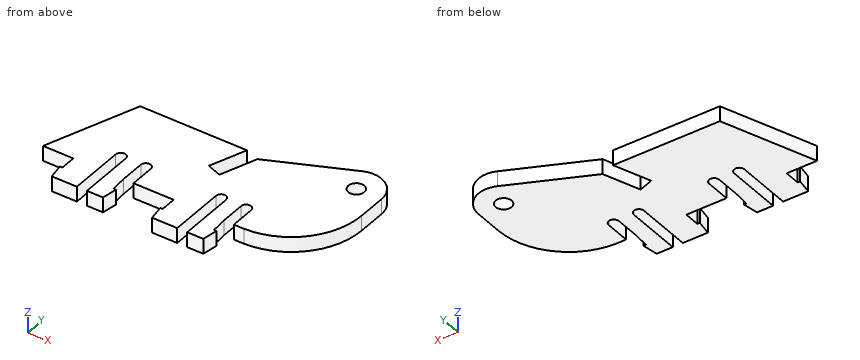
from build123d import *

# Parameters (mm, degrees)
SKETCH1_R           = 1.5875
BOSS_EXTRUDE1_DEPTH = 3
TABS_DEPTH          = 3
TAB_RELIEF_REACH    = 195.217


with BuildPart() as part:
    # Sketch1 → Boss-Extrude1 (new body)
    with BuildSketch(Plane.XY):
        with BuildLine():
            Line((-44.534658728, 169.908603759), (-60.444091073, 162.821196289))
            Line((-60.444091073, 162.821196289), (-63.031525128, 155.712279649))
            Line((-63.031525128, 155.712279649), (-65.85060299, 156.738340079))
            Line((-65.85060299, 156.738340079), (-63.263168935, 163.847256719))
            Line((-63.263168935, 163.847256719), (-84.546724385, 163.847256719))
            Line((-84.546724385, 163.847256719), (-91.147316237, 145.712279649))
            Line((-91.147316237, 145.712279649), (-51.5, 145.712279649))
            ThreePointArc((-51.5, 145.712279649), (-41.600505063, 149.812784712), (-37.5, 159.712279649))
            Line((-37.5, 159.712279649), (-37.5, 165.341310922))
            ThreePointArc((-37.5, 165.341310922), (-39.777252641, 169.534954543), (-44.534658728, 169.908603759))
        make_face()
        with Locations((-42.5, 165.341310922)):
            Circle(SKETCH1_R, mode=Mode.SUBTRACT)
    extrude(amount=BOSS_EXTRUDE1_DEPTH)

    # Sketch3 → tabs (add)
    with BuildSketch(Plane(origin=(0, 0, 0), x_dir=(-1, 0, 0), z_dir=(0, 0, -1))):
        with BuildLine():
            Line((54.9, 142.612279649), (55.1, 145.712279649))
            Line((55.1, 145.712279649), (55.1, 150.612279649))
            ThreePointArc((55.1, 150.612279649), (54.1, 151.612279649), (53.1, 150.612279649))
            Line((53.1, 150.612279649), (53.1, 145.712279649))
            Line((53.1, 145.712279649), (51.1, 145.712279649))
            Line((51.1, 145.712279649), (51.1, 152.712279649))
            Line((51.1, 152.712279649), (67.1, 152.712279649))
            Line((67.1, 152.712279649), (67.1, 145.712279649))
            Line((67.1, 145.712279649), (65.1, 145.712279649))
            Line((65.1, 145.712279649), (65.1, 142.612279649))
            Line((65.1, 142.612279649), (65.6, 142.612279649))
            Line((65.6, 142.612279649), (65.1, 139.612279649))
            Line((65.1, 139.612279649), (60.1, 139.612279649))
            Line((60.1, 139.612279649), (60.1, 150.612279649))
            ThreePointArc((60.1, 150.612279649), (59.1, 151.612279649), (58.1, 150.612279649))
            Line((58.1, 150.612279649), (58.1, 139.612279649))
            Line((58.1, 139.612279649), (54.9, 139.612279649))
            Line((54.9, 139.612279649), (54.4, 142.612279649))
            Line((54.4, 142.612279649), (54.9, 142.612279649))
        make_face()
        with BuildLine():
            Line((74.9, 142.612279649), (75.1, 145.712279649))
            Line((75.1, 145.712279649), (75.1, 150.612279649))
            ThreePointArc((75.1, 150.612279649), (74.1, 151.612279649), (73.1, 150.612279649))
            Line((73.1, 150.612279649), (73.1, 145.712279649))
            Line((73.1, 145.712279649), (71.1, 145.712279649))
            Line((71.1, 145.712279649), (71.1, 152.712279649))
            Line((71.1, 152.712279649), (87.1, 152.712279649))
            Line((87.1, 152.712279649), (87.1, 145.712279649))
            Line((87.1, 145.712279649), (85.1, 145.712279649))
            Line((85.1, 145.712279649), (85.1, 142.612279649))
            Line((85.1, 142.612279649), (85.6, 142.612279649))
            Line((85.6, 142.612279649), (85.1, 139.612279649))
            Line((85.1, 139.612279649), (80.1, 139.612279649))
            Line((80.1, 139.612279649), (80.1, 150.612279649))
            ThreePointArc((80.1, 150.612279649), (79.1, 151.612279649), (78.1, 150.612279649))
            Line((78.1, 150.612279649), (78.1, 139.612279649))
            Line((78.1, 139.612279649), (74.9, 139.612279649))
            Line((74.9, 139.612279649), (74.4, 142.612279649))
            Line((74.4, 142.612279649), (74.9, 142.612279649))
        make_face()
    extrude(amount=-TABS_DEPTH)

    # Sketch4 → tab relief (cut, up to next)
    with BuildSketch(Plane(origin=(0, 0, 0), x_dir=(-1, 0, 0), z_dir=(0, 0, -1)), mode=Mode.PRIVATE) as tab_relief_sk1:
        with BuildLine():
            Line((55.1, 145.712279649), (55.1, 150.612279649))
            ThreePointArc((55.1, 150.612279649), (54.1, 151.612279649), (53.1, 150.612279649))
            Line((53.1, 150.612279649), (53.1, 145.712279649))
            Line((53.1, 145.712279649), (55.1, 145.712279649))
        make_face()
    tab_relief_tool1 = extrude(tab_relief_sk1.sketch, amount=-TAB_RELIEF_REACH, mode=Mode.PRIVATE) & part.part
    # Sketch4 → tab relief (cut, up to next)
    with BuildSketch(Plane(origin=(0, 0, 0), x_dir=(-1, 0, 0), z_dir=(0, 0, -1)), mode=Mode.PRIVATE) as tab_relief_sk2:
        with BuildLine():
            Line((75.1, 145.712279649), (75.1, 150.612279649))
            ThreePointArc((75.1, 150.612279649), (74.1, 151.612279649), (73.1, 150.612279649))
            Line((73.1, 150.612279649), (73.1, 145.712279649))
            Line((73.1, 145.712279649), (75.1, 145.712279649))
        make_face()
    tab_relief_tool2 = extrude(tab_relief_sk2.sketch, amount=-TAB_RELIEF_REACH, mode=Mode.PRIVATE) & part.part
    # Sketch4 → tab relief (cut, up to next)
    with BuildSketch(Plane(origin=(0, 0, 0), x_dir=(-1, 0, 0), z_dir=(0, 0, -1)), mode=Mode.PRIVATE) as tab_relief_sk3:
        with BuildLine():
            Line((58.1, 150.612279649), (58.1, 145.712279649))
            Line((58.1, 145.712279649), (60.1, 145.712279649))
            Line((60.1, 145.712279649), (60.1, 150.612279649))
            ThreePointArc((60.1, 150.612279649), (59.1, 151.612279649), (58.1, 150.612279649))
        make_face()
    tab_relief_tool3 = extrude(tab_relief_sk3.sketch, amount=-TAB_RELIEF_REACH, mode=Mode.PRIVATE) & part.part
    # Sketch4 → tab relief (cut, up to next)
    with BuildSketch(Plane(origin=(0, 0, 0), x_dir=(-1, 0, 0), z_dir=(0, 0, -1)), mode=Mode.PRIVATE) as tab_relief_sk4:
        with BuildLine():
            Line((78.1, 150.612279649), (78.1, 145.712279649))
            Line((78.1, 145.712279649), (80.1, 145.712279649))
            Line((80.1, 145.712279649), (80.1, 150.612279649))
            ThreePointArc((80.1, 150.612279649), (79.1, 151.612279649), (78.1, 150.612279649))
        make_face()
    tab_relief_tool4 = extrude(tab_relief_sk4.sketch, amount=-TAB_RELIEF_REACH, mode=Mode.PRIVATE) & part.part
    add(tab_relief_tool1.solids().sort_by_distance((-54.1, 148.55936, 0))[0], mode=Mode.SUBTRACT)
    add(tab_relief_tool2.solids().sort_by_distance((-74.1, 148.55936, 0))[0], mode=Mode.SUBTRACT)
    add(tab_relief_tool3.solids().sort_by_distance((-59.1, 148.55936, 0))[0], mode=Mode.SUBTRACT)
    add(tab_relief_tool4.solids().sort_by_distance((-79.1, 148.55936, 0))[0], mode=Mode.SUBTRACT)


solid = part.part
Can you work these out from the model? Positions are in its coordinate system, mm. Coordinates: 2 decimals unless noted, no trailing zeros. Loops run counter-clockwise (first coordinate to the right, second up) from the corner with the lowest first, then second, coordinate; pieces in that order, holes last. Notation, with made-up numbers: (15.5, 17.5) - (57.5, 17.5) arc R10 ccw to (57.5, 26.5) - close; hole circle Ø9 at (65, 34). An arc over 180 degrees is marked (long way). Answer as a JSON object with one key per item and string values. Group by question number.
Item 1: If we section it at C-C (x = -67.5): List the corners of the cut face in (y, z) for me, plus the area to 3 significant figures.
Item 2: For pin 1 (1.5 mm diameter, centred on y = 146.5, z = 1, fed in from +X); pin 2 (1.5 mm diameter, centred on y = 143.5, z = 1.5, fed in from -X); pin 3 (1 mm diameter, centred on x = -52, z = 1, fed in from -Y), each with a flat end and sliding along its axis, tell me the tip position at first contact or that it passes through.
Item 3: If we section it at A-A (x = -42.5): List the corners of the cut face in (y, z) for me, plus the area to 3 significant figures.
Item 4: If we section it at B-B (y = 147): List the corners of the cut face in (x, z) for me.
Item 5: If we section it at D-D (y = 154): List the corners of the cut face in (x, z) for me.
Item 6: If I drill on L1, parallel to X at y = 145.5, z = 2.5; L2, parallel to X at y = 151.5, z = 2.8; L3, parallel to Y at x = -72, z = 1.7, over which ranges is the centre line in solid material (lowest first)? Write a range as from..to.
Returned:
{
 "1": {"outline": "(145.71, 0) - (163.85, 0) - (163.85, 3) - (145.71, 3) - close", "area": "54.4 mm²"},
 "2": {"pin 1": "stops at x = -45.12", "pin 2": "stops at x = -85.1", "pin 3": "stops at y = 145.71"},
 "3": {"outline": "(148.99, 0) - (163.75, 0) - (163.75, 3) - (148.99, 3) - close; (166.93, 0) - (170.34, 0) - (170.34, 3) - (166.93, 3) - close", "area": "54.5 mm²"},
 "4": {"outline": "(-90.68, 0) - (-80.1, 0) - (-80.1, 3) - (-90.68, 3) - close; (-78.1, 0) - (-75.1, 0) - (-75.1, 3) - (-78.1, 3) - close; (-73.1, 0) - (-60.1, 0) - (-60.1, 3) - (-73.1, 3) - close; (-58.1, 0) - (-55.1, 0) - (-55.1, 3) - (-58.1, 3) - close; (-53.1, 0) - (-45.64, 0) - (-45.64, 3) - (-53.1, 3) - close"},
 "5": {"outline": "(-88.13, 0) - (-38.72, 0) - (-38.72, 3) - (-88.13, 3) - close"},
 "6": {"L1": "x = -85.1..-80.1, -78.1..-75.09, -65.1..-60.1, -58.1..-55.09", "L2": "x = -89.04..-79.56, -78.64..-74.56, -73.64..-59.56, -58.64..-54.56, -53.64..-40.16", "L3": "y = 145.71..163.85"}
}
